Check sheet for the modelled part. Datum: model origin and axes. Units: mm. Round coordinates to 2 decimals unless told otherwise and drop trailing zeros. Loops run counter-clockwise (first coordinate to the right, second up) from the corner with the lowest first, then second, coordinate; pieces in that order, holes last. Notation, with made-up numbers: M -40,0.5 L -31,0.5 A20 ccw -31,18.5 Z; hole C 2.5,71.25 d1. An arc over 180 degrees is marked long. Write item = value, one per line. Start each with the question number.
(1) Cross-section at D-D on y = -4.25. Record the boundary of the cut face in (x, z).
(2) Cross-section at B-B on x = 0. Record the boundary of the cut face in (y, z).
(3) Cross-section at C-C on z = 38.5. Record the boundary of the cut face in (x, y).
(4) Scan lines: L1, parallel to Z at x = -5, y = 3.5; L2, parallel to Y at x = 0, z = 13.5; L3, parallel to X at y = 1.5, z = 84. Record each from-to range of solid material in increasing order. Write a range as from..to.
(5) Cross-section at A-A on z = 87.5. Record the boundary of the cut face in (x, y), plus the area to 3 significant figures.
(6) Go/stop test with flat-tipped pins: P1, Ø5, axis at x = -4, z = 74.5, coming from the -Y side; P2, Ø2, axis at y = -3.5, z = 35, coming from the +X side; P3, Ø1.5, axis at x = 0, y = 1, coming from the +Z side; P4, Ø2, axis at x = 5.5, z = 65, coming from the -Y side. Record where each tip stops, or that it passes through.
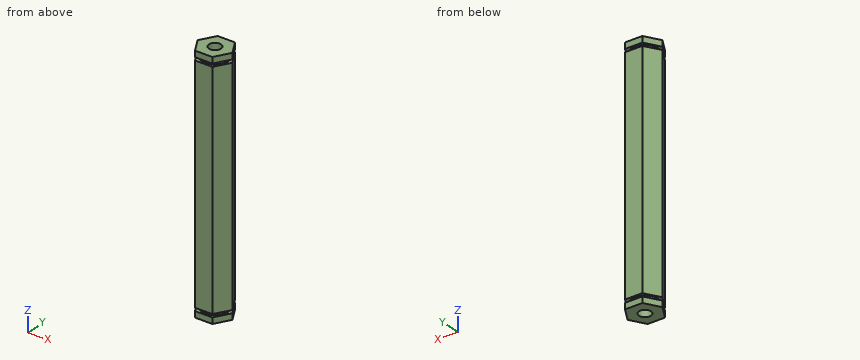
from build123d import *

# Parameters (mm, degrees)
BOSS_EXTRUDE1_DEPTH = 103.1875
SKETCH2_R           = 9.90966703
SKETCH2_R_2         = 5.635297177
CUT_EXTRUDE1_DEPTH  = 1.27
SKETCH3_R           = 2.54
CUT_EXTRUDE2_DEPTH  = 25.4
SKETCH4_R           = 26.134229338
SKETCH4_R_2         = 5.635297177
CUT_EXTRUDE3_DEPTH  = 1.27
SKETCH5_R           = 2.54
CUT_EXTRUDE4_DEPTH  = 25.4


with BuildPart() as part:
    # Sketch1 → Boss-Extrude1 (new body)
    with BuildSketch(Plane.XY):
        Polygon((7.332348419, 0), (3.666174209, 6.35), (-3.666174209, 6.35), (-7.332348419, 0), (-3.666174209, -6.35), (3.666174209, -6.35), align=None)
    extrude(amount=BOSS_EXTRUDE1_DEPTH)

    # Sketch2 → Cut-Extrude1 (cut)
    with BuildSketch(Plane.XY.offset(2.54)):
        Circle(SKETCH2_R)
        Circle(SKETCH2_R_2, mode=Mode.SUBTRACT)
    extrude(amount=CUT_EXTRUDE1_DEPTH, mode=Mode.SUBTRACT)

    # Sketch3 → Cut-Extrude2 (cut)
    with BuildSketch(Plane(origin=(0, 0, 0), x_dir=(-1, 0, 0), z_dir=(0, 0, -1))):
        Circle(SKETCH3_R)
    extrude(amount=-CUT_EXTRUDE2_DEPTH, mode=Mode.SUBTRACT)

    # Sketch4 → Cut-Extrude3 (cut)
    with BuildSketch(Plane.XY.offset(100.6475)):
        Circle(SKETCH4_R)
        Circle(SKETCH4_R_2, mode=Mode.SUBTRACT)
    extrude(amount=-CUT_EXTRUDE3_DEPTH, mode=Mode.SUBTRACT)

    # Sketch5 → Cut-Extrude4 (cut)
    with BuildSketch(Plane.XY.offset(103.1875)):
        Circle(SKETCH5_R)
    extrude(amount=-CUT_EXTRUDE4_DEPTH, mode=Mode.SUBTRACT)


solid = part.part
Result:
q1.outline = M -4.88,0 L 4.88,0 L 4.88,2.54 L 3.7,2.54 L 3.7,3.81 L 4.88,3.81 L 4.88,99.38 L 3.7,99.38 L 3.7,100.65 L 4.88,100.65 L 4.88,103.19 L -4.88,103.19 L -4.88,100.65 L -3.7,100.65 L -3.7,99.38 L -4.88,99.38 L -4.88,3.81 L -3.7,3.81 L -3.7,2.54 L -4.88,2.54 Z
q2.outline = M -6.35,0 L -2.54,0 L -2.54,25.4 L 2.54,25.4 L 2.54,0 L 6.35,0 L 6.35,2.54 L 5.64,2.54 L 5.64,3.81 L 6.35,3.81 L 6.35,99.38 L 5.64,99.38 L 5.64,100.65 L 6.35,100.65 L 6.35,103.19 L 2.54,103.19 L 2.54,77.79 L -2.54,77.79 L -2.54,103.19 L -6.35,103.19 L -6.35,100.65 L -5.64,100.65 L -5.64,99.38 L -6.35,99.38 L -6.35,3.81 L -5.64,3.81 L -5.64,2.54 L -6.35,2.54 Z
q3.outline = M -7.33,0 L -3.67,-6.35 L 3.67,-6.35 L 7.33,0 L 3.67,6.35 L -3.67,6.35 Z
q4.L1 = 0..2.54, 3.81..99.38, 100.65..103.19
q4.L2 = -6.35..-2.54, 2.54..6.35
q4.L3 = -6.47..-2.05, 2.05..6.47
q5.outline = M -7.33,0 L -3.67,-6.35 L 3.67,-6.35 L 7.33,0 L 3.67,6.35 L -3.67,6.35 Z; hole C 0,0 d5.08
q5.area = 119 mm^2
q6.P1 = -6.35
q6.P2 = 5.89
q6.P3 = 77.79
q6.P4 = -4.91
